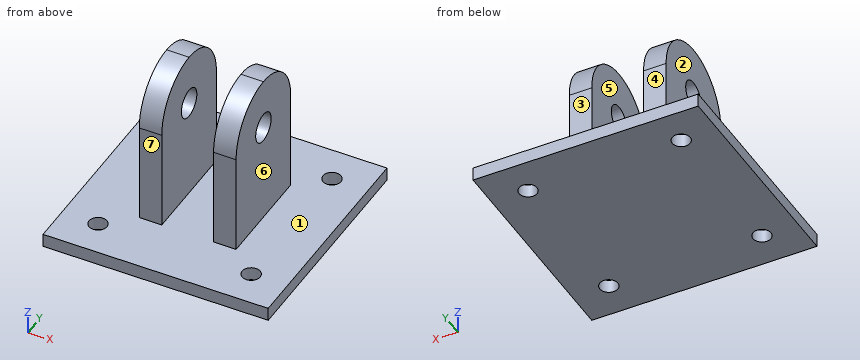
```python
from build123d import *

# Parameters (mm, degrees)
F0_W     = 50
F0_H     = 50
F1_DEPTH = 3
F3_DEPTH = 34
F4_R     = 11.49999
F6_D     = 6.5
F8_D     = 4
F8_DEPTH = 15
F8_TIP   = 1.2017212381


# Not quite as in the source:
# - a fillet or chamfer is up to 0.001 mm smaller than in the source, because OpenCascade refuses the exact size


with BuildPart() as f1:
    # F0 (on Top) → F1 (new body)
    with BuildSketch(Plane.XY):
        Rectangle(F0_W, F0_H)
    extrude(amount=F1_DEPTH)

    # F2 (on face) → F3 (join)
    with BuildSketch(Plane.XY.offset(3)):
        Polygon((5.74977943, 11.5), (5.74977943, 0), (5.74977943, -11.4999999979), (10.74977943, -11.4999999979), (10.74977943, 2.1e-09), (10.74977943, 11.5), align=None)
        Polygon((-5.75022057, -11.4999999979), (-5.75, 0), (-5.74977943, 11.5000000021), (-10.75022057, 11.5000000021), (-10.75022057, 2.1e-09), (-10.75022057, -11.4999999979), align=None)
    extrude(amount=F3_DEPTH)

    # F4 (radius 11.5 in the source; OpenCascade refuses exactly that, so slightly less here)
    f4_edges = [f1.edges().sort_by_distance(p)[0] for p in [
        (-8.250221, -11.5, 37),
        (8.249779, -11.5, 37),
        (8.249779, 11.5, 37),
        (-8.25, 11.5, 37),
    ]]
    fillet(f4_edges, radius=F4_R)

    # F6 (through all)
    with Locations(Plane(origin=(-10.75022057, 0, 0), x_dir=(0, -1, 0), z_dir=(-1, 0, 0))):
        with Locations((-2.1e-09, 25.5)):
            Hole(F6_D / 2)

    # F8
    with Locations(Plane.XY.offset(3)):
        with Locations((-17, 17), (17, 17), (17, -17), (-17, -17)):
            Hole(F8_D / 2, depth=F8_DEPTH)
            with Locations((0, 0, -(F8_DEPTH + F8_TIP / 2))):  # 118° drill point
                Cone(0, F8_D / 2, F8_TIP, mode=Mode.SUBTRACT)


solid = f1.part
```
Geometry check sheet. Reference: the model listing, model coordinates, mm. Face numbers are marked on the shaded views. A direction names the side the tool comes from. Coordinates: 2 decimals unless noted, no trailing zeros. Order: outer loops, then holes, each group sorted by start corner. A loop starts at its lowest first (then second) coordinate and runs counter-clockwise, first axis right, second up. Notation, with made-up numbers: (-16, 22.5) - (37, 22.5) arc R12 ccw to (37, 33.5) - close; hole circle Ø2 at (14, 24). An arc over 180 degrees is marked (long way). Answer as a JSON object with one key per item and string values. Group by question number.
Item 1: Sectioned sample at B-B, the plane z = 4.5. Record the cut outline in (x, y), and give its area (3 significant figures).
Item 2: Sectioned sample at A-A, the plane y = 17. Record the cut outline in (x, z), and give its area (3 significant figures).
Item 3: Tool access check on the marked faces 4, 5, 6 and 7. Record the directions out of +Z, -Z, +X, -X, +Y, -Y that give a thin tool (end or side, any length) a straight path to the whole face; none if there is none.
Item 4: Scan lines: probe 1 along Y at (x, z) = (17, 2.45); probe 2 along Z at (x, y) = (-7, 0); probe 3 along X at (y, z) = (-5, 15.5). Record each from-to range of solid material in increasing order.
Item 5: Depth check by flat-ended pin: pin 1 Ø10 at (y, z) = (-11.5, 16) entering from -X; pin 2 Ø7 at (y, z) = (0, 21) entering from +X; pin 3 Ø10 at (x, z) = (-7, 25) entering from +Y. Enter the tip coordinate at first touch or a pass-through.
Item 6: Draft check along X on the marked faces 1, 2 and 3. Enter one of: +X half, -X half, draft (parallel to the pull), parting line (faces both ways), or undercut.
Resolved:
{
 "1": {"outline": "(-10.75, -11.5) - (-5.75, -11.5) - (-5.75, 11.5) - (-10.75, 11.5) - close; (5.75, -11.5) - (10.75, -11.5) - (10.75, 11.5) - (5.75, 11.5) - close", "area": "230 mm^2"},
 "2": {"outline": "(-25, 0) - (-19, 0) - (-19, 3) - (-25, 3) - close; (-15, 0) - (15, 0) - (15, 3) - (-15, 3) - close; (19, 0) - (25, 0) - (25, 3) - (19, 3) - close", "area": "126 mm^2"},
 "3": {"face 4": "+Z, +X, -X, +Y", "face 5": "+Z, +Y, -Y", "face 6": "+Z, +X, +Y, -Y", "face 7": "+Z, +X, -X, -Y"},
 "4": {"probe 1": "-25 to -19, -15 to 15, 19 to 25", "probe 2": "0 to 22.25, 28.75 to 37", "probe 3": "-10.75 to -5.75, 5.75 to 10.75"},
 "5": {"pin 1": "x = -10.75", "pin 2": "x = 10.75", "pin 3": "y = 11.5"},
 "6": {"face 1": "undercut", "face 2": "-X half", "face 3": "draft"}
}
